Can you work these out from the model? Positions are in its coordinate system, mm. Face numbers are marked on the shaded views. A direction names the side the tool comes from. Coordinates: 2 decimals unless noted, no trailing zeros. Order: outer loops, then holes, each group sorted by start corner. A loop starts at its lowest first (then second) coordinate and runs counter-clockwise, first axis right, second up. Notation, with made-up numbers: (9, 77) - (53, 77) arc R23 ccw to (53, 99) - close; hole circle Ø1 at (86.25, 38.25). An arc over 180 degrees is marked (long way). Return JSON: item names as keys, results as strings. Group by question number.
1) If I drill on line 1 along Y through (x, z) = (59.1, 66); line 2 along Z through (x, y) = (58.6, -20) (3 decimals); line 3 along Y through (x, z) = (60, 68), over which ranges is the centre line in solid material (lowest first)?
2) Which directions (+Z, -Z, +X, -X, +Y, -Y) give clear straight access to the entire face, cutting with the end or side of a thin tool? Please do the marked faces 1, 2 and 3.
3) Imagine slicing it at A-A (y = -20). Write out the boundary of the cut face in (x, z) (3 decimals), and give its area (3 significant figures).
4) If we mould it in two halves opening along Y, with no side actions, what happens to the marked faces 4, 5 and 6? For each: pulls with the +Y half, pulls with the -Y half, needs draft (parallel to the pull), parting line crosses it, or undercut.
5) Imagine slicing it at B-B (z = 66). Write out the boundary of the cut face in (x, y), and give its area (3 significant figures).
6) For pin 1 Ø1.6 at (x, z) = (56.5, 79) entering from -Y; pin 2 Ø0.9 at (x, z) = (58.5, 57.5) entering from -Y; pin 3 Ø2 at (y, z) = (-15, 63) entering from -X; pin 4 Ø2 at (x, y) = (56, -21) entering from -Z, each with a flat end and sliding along its axis, tell me the tip position at first contact or that it passes through.
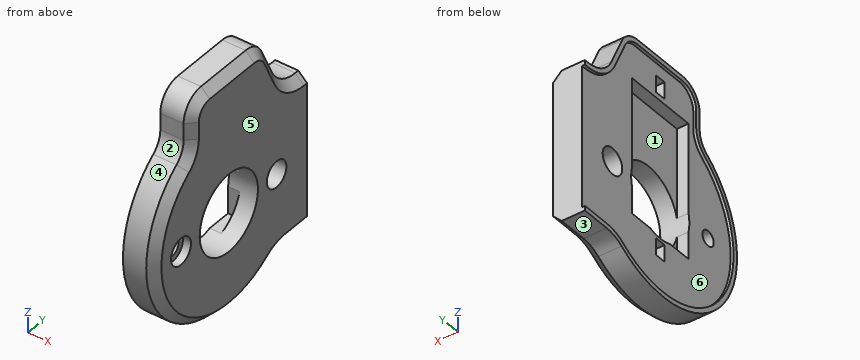
```python
from build123d import *

# Parameters (mm, degrees)
BOSS_EXTRUDE1_START  = 55.1
BOSS_EXTRUDE1_DEPTH  = 5.5
BOSS_EXTRUDE2_START  = 55
BOSS_EXTRUDE2_DEPTH  = 0.6
CHAMFER1_SIZE        = 1.5
BOSS_EXTRUDE3_START  = 55.875
SKETCH3_W            = 4.1
SKETCH3_H            = 2
BOSS_EXTRUDE3_DEPTH  = 2.9
BOSS_EXTRUDE4_START  = 84.025
SKETCH4_W            = 4.1
SKETCH4_H            = 2
BOSS_EXTRUDE4_DEPTH  = 2.9
BOSS_EXTRUDE5_START  = 59.7
SKETCH5_W            = 2.1
SKETCH5_H            = 13
BOSS_EXTRUDE5_DEPTH  = 23.4
BOSS_EXTRUDE6_START  = 55.5
SKETCH6_R            = 6.7
BOSS_EXTRUDE6_DEPTH  = 5.6
BOSS_EXTRUDE7_START  = 55.5
SKETCH7_R            = 2.25
BOSS_EXTRUDE7_DEPTH  = 5.6
BOSS_EXTRUDE8_START  = 59.2
SKETCH8_R            = 2.3
BOSS_EXTRUDE8_DEPTH  = 1.9
BOSS_EXTRUDE9_START  = 55.5
SKETCH9_R            = 1.3
BOSS_EXTRUDE9_DEPTH  = 3.75
BOSS_EXTRUDE10_START = 26
SKETCH10_W           = 30
SKETCH10_H           = 62
BOSS_EXTRUDE10_DEPTH = 80


with BuildPart() as part:
    # Sketch1 → Boss-Extrude1 (new body)
    with BuildSketch(Plane(origin=(0, 0, 0), x_dir=(0, 0, -1), z_dir=(1, 0, 0)).offset(BOSS_EXTRUDE1_START)):
        with BuildLine():
            Line((-53, 3.337121701), (-53, -7.038518603))
            ThreePointArc((-53, -7.038518603), (-52.733198515, -8.807822077), (-51.956521739, -10.41977462))
            ThreePointArc((-51.956521739, -10.41977462), (-56.18950583, -33.883594784), (-79.719936005, -30.038095238))
            ThreePointArc((-79.719936005, -30.038095238), (-81.138131249, -28.832955071), (-82.948156242, -28.4))
            Line((-82.948156242, -28.4), (-85.85, -28.4))
            ThreePointArc((-85.85, -28.4), (-88.678427125, -27.228427125), (-89.85, -24.4))
            Line((-89.85, -24.4), (-89.85, -14.139667829))
            ThreePointArc((-89.85, -14.139667829), (-89.226856881, -11.995644133), (-87.551581196, -10.519637244))
            Line((-87.551581196, -10.519637244), (-82.447628205, -8.120544133))
            ThreePointArc((-82.447628205, -8.120544133), (-79.934714679, -5.9065338), (-79, -2.690498257))
            Line((-79, -2.690498257), (-79, 3.337121701))
            ThreePointArc((-79, 3.337121701), (-79.321091654, 5.273613374), (-80.25, 7.002841276))
            ThreePointArc((-80.25, 7.002841276), (-66, 36), (-51.75, 7.002841276))
            ThreePointArc((-51.75, 7.002841276), (-52.678908346, 5.273613374), (-53, 3.337121701))
        make_face()
    extrude(amount=BOSS_EXTRUDE1_DEPTH)


with BuildPart() as body_2:
    # Sketch2 → Boss-Extrude2 (new body)
    with BuildSketch(Plane(origin=(0, 0, 0), x_dir=(0, 0, -1), z_dir=(1, 0, 0)).offset(BOSS_EXTRUDE2_START)):
        with BuildLine():
            Line((-53.8, 3.337121701), (-53.8, -7.038518603))
            ThreePointArc((-53.8, -7.038518603), (-53.497624984, -9.043729207), (-52.617391304, -10.870608755))
            ThreePointArc((-52.617391304, -10.870608755), (-56.651176143, -33.230249147), (-79.074291958, -29.565714286))
            ThreePointArc((-79.074291958, -29.565714286), (-80.77612625, -28.119546085), (-82.948156242, -27.6))
            Line((-82.948156242, -27.6), (-85.85, -27.6))
            ThreePointArc((-85.85, -27.6), (-88.1127417, -26.6627417), (-89.05, -24.4))
            Line((-89.05, -24.4), (-89.05, -14.139667829))
            ThreePointArc((-89.05, -14.139667829), (-88.551485505, -12.424448872), (-87.211264957, -11.243643361))
            Line((-87.211264957, -11.243643361), (-82.107311966, -8.84455025))
            ThreePointArc((-82.107311966, -8.84455025), (-79.259343303, -6.335338539), (-78.2, -2.690498257))
            Line((-78.2, -2.690498257), (-78.2, 3.337121701))
            ThreePointArc((-78.2, 3.337121701), (-78.563903875, 5.531812264), (-79.616666667, 7.491603886))
            ThreePointArc((-79.616666667, 7.491603886), (-66, 35.2), (-52.383333333, 7.491603886))
            ThreePointArc((-52.383333333, 7.491603886), (-53.436096125, 5.531812264), (-53.8, 3.337121701))
        make_face()
    extrude(amount=BOSS_EXTRUDE2_DEPTH)


with BuildPart() as part_1:
    add(part.part)

    # Combine1: cut body 2
    add(body_2.part, mode=Mode.SUBTRACT)

    # Chamfer1
    chamfer1_edges = [part_1.edges().sort_by_distance(p)[0] for p in [
        (60.6, -5.9065338, 79.934714679),
        (60.6, -9.320090689, 84.999604701),
        (60.6, -11.995644133, 89.226856881),
        (60.6, -19.269833914, 89.85),
        (60.6, -27.228427125, 88.678427125),
        (60.6, -28.4, 84.399078121),
        (60.6, -28.832955071, 81.138131249),
        (60.6, -33.883594784, 56.18950583),
        (60.6, -8.807822077, 52.733198515),
        (60.6, -1.850698451, 53),
        (60.6, 5.273613374, 79.321091654),
        (60.6, 5.273613374, 52.678908346),
        (60.6, 36, 66),
        (60.6, 0.323311722, 79),
    ]]
    chamfer(chamfer1_edges, length=CHAMFER1_SIZE)


with BuildPart() as body_2_2:
    # Sketch3 → Boss-Extrude3 (new body)
    with BuildSketch(Plane.XY.offset(BOSS_EXTRUDE3_START)):
        with Locations((57.55, -20)):
            Rectangle(SKETCH3_W, SKETCH3_H)
    extrude(amount=BOSS_EXTRUDE3_DEPTH)


with BuildPart() as part_2:
    add(part_1.part)

    # Combine2: cut body 2 2
    add(body_2_2.part, mode=Mode.SUBTRACT)


with BuildPart() as body_2_3:
    # Sketch4 → Boss-Extrude4 (new body)
    with BuildSketch(Plane.XY.offset(BOSS_EXTRUDE4_START)):
        with Locations((57.55, -20)):
            Rectangle(SKETCH4_W, SKETCH4_H)
    extrude(amount=BOSS_EXTRUDE4_DEPTH)


with BuildPart() as part_3:
    add(part_2.part)

    # Combine3: cut body 2 3
    add(body_2_3.part, mode=Mode.SUBTRACT)


with BuildPart() as body_2_4:
    # Sketch5 → Boss-Extrude5 (new body)
    with BuildSketch(Plane.XY.offset(BOSS_EXTRUDE5_START)):
        with Locations((56.55, -20)):
            Rectangle(SKETCH5_W, SKETCH5_H)
    extrude(amount=BOSS_EXTRUDE5_DEPTH)


with BuildPart() as part_4:
    add(part_3.part)

    # Combine4: cut body 2 4
    add(body_2_4.part, mode=Mode.SUBTRACT)


with BuildPart() as body_2_5:
    # Sketch6 → Boss-Extrude6 (new body)
    with BuildSketch(Plane(origin=(0, 0, 0), x_dir=(0, 0, -1), z_dir=(1, 0, 0)).offset(BOSS_EXTRUDE6_START)):
        with Locations((-66, -20)):
            Circle(SKETCH6_R)
    extrude(amount=BOSS_EXTRUDE6_DEPTH)


with BuildPart() as part_5:
    add(part_4.part)

    # Combine5: cut body 2 5
    add(body_2_5.part, mode=Mode.SUBTRACT)


with BuildPart() as body_2_6:
    # Sketch7 → Boss-Extrude7 (new body)
    with BuildSketch(Plane(origin=(0, 0, 0), x_dir=(0, 0, -1), z_dir=(1, 0, 0)).offset(BOSS_EXTRUDE7_START)):
        with Locations((-66, -9)):
            Circle(SKETCH7_R)
    extrude(amount=BOSS_EXTRUDE7_DEPTH)


with BuildPart() as part_6:
    add(part_5.part)

    # Combine6: cut body 2 6
    add(body_2_6.part, mode=Mode.SUBTRACT)


with BuildPart() as body_2_7:
    # Sketch8 → Boss-Extrude8 (new body)
    with BuildSketch(Plane(origin=(0, 0, 0), x_dir=(0, 0, -1), z_dir=(1, 0, 0)).offset(BOSS_EXTRUDE8_START)):
        with Locations((-66, -31)):
            Circle(SKETCH8_R)
    extrude(amount=BOSS_EXTRUDE8_DEPTH)


with BuildPart() as part_7:
    add(part_6.part)

    # Combine7: cut body 2 7
    add(body_2_7.part, mode=Mode.SUBTRACT)


with BuildPart() as body_2_8:
    # Sketch9 → Boss-Extrude9 (new body)
    with BuildSketch(Plane(origin=(0, 0, 0), x_dir=(0, 0, -1), z_dir=(1, 0, 0)).offset(BOSS_EXTRUDE9_START)):
        with Locations((-66, -31)):
            Circle(SKETCH9_R)
    extrude(amount=BOSS_EXTRUDE9_DEPTH)


with BuildPart() as part_8:
    add(part_7.part)

    # Combine8: cut body 2 8
    add(body_2_8.part, mode=Mode.SUBTRACT)


with BuildPart() as body_2_9:
    # Sketch10 → Boss-Extrude10 (new body)
    with BuildSketch(Plane.XY.offset(BOSS_EXTRUDE10_START)):
        with Locations((55, 29)):
            Rectangle(SKETCH10_W, SKETCH10_H)
    extrude(amount=BOSS_EXTRUDE10_DEPTH)


with BuildPart() as part_9:
    add(part_8.part)

    # Combine9: cut body 2 9
    add(body_2_9.part, mode=Mode.SUBTRACT)


solid = part_9.part
```
Calculated:
{
 "1": {"line 1": "-37 to -32.3, -29.7 to -26.7, -13.3 to -11.25, -6.75 to -2", "line 2": "49 to 55.875, 58.775 to 59.3, 72.7 to 84.025, 86.925 to 89.85", "line 3": "-35.98 to -32.14, -29.86 to -26.39, -13.61 to -10.03, -7.97 to -2"},
 "2": {"face 1": "-X", "face 2": "+Z, +X, -X, -Y", "face 3": "-Z, +X, -X, +Y"},
 "3": {"outline": "(55.1, 49) - (59.1, 49) - (60.6, 50.5) - (60.6, 59.3) - (55.6, 59.3) - (55.6, 58.775) - (59.6, 58.775) - (59.6, 55.875) - (55.6, 55.875) - (55.6, 49.8) - (55.1, 49.8) - close; (55.1, 89.05) - (55.6, 89.05) - (55.6, 86.925) - (59.6, 86.925) - (59.6, 84.025) - (55.6, 84.025) - (55.6, 83.1) - (57.6, 83.1) - (57.6, 72.7) - (60.6, 72.7) - (60.6, 88.35) - (59.1, 89.85) - (55.1, 89.85) - close", "area": "91.8 mm2"},
 "4": {"face 4": "parting line crosses it", "face 5": "needs draft", "face 6": "undercut"},
 "5": {"outline": "(55.1, -37) - (59.1, -37) - (60.6, -35.5) - (60.6, -33.3) - (59.2, -33.3) - (59.2, -32.3) - (55.6, -32.3) - (55.6, -36.2) - (55.1, -36.2) - close; (55.6, -29.7) - (59.2, -29.7) - (59.2, -28.7) - (60.6, -28.7) - (60.6, -26.7) - (55.6, -26.7) - close; (55.6, -13.3) - (60.6, -13.3) - (60.6, -11.25) - (55.6, -11.25) - close; (55.6, -6.75) - (60.6, -6.75) - (60.6, -2) - (55.6, -2) - close", "area": "69.0 mm2"},
 "6": {"pin 1": "y = -31.84", "pin 2": "y = -34.97", "pin 3": "x = 57.6", "pin 4": "z = 49"}
}
